```python
from build123d import *

# Parameters (mm, degrees)
SKETCH3_W           = 25.4
SKETCH3_H           = 12.7
SKETCH3_W_2         = 127
BOSS_EXTRUDE1_DEPTH = 6.35
FILLET1_R           = 7.62
SKETCH5_R           = 3.175
CUT_EXTRUDE2_DEPTH  = 13.7


with BuildPart() as part:
    # Sketch3 → Boss-Extrude1 (new body, symmetric)
    with BuildSketch(Plane(origin=(0, 0, 0), x_dir=(0, 0, -1), z_dir=(1, 0, 0))):
        with Locations((88.9, 0)):
            Rectangle(SKETCH3_W, SKETCH3_H)
        Polygon((76.2, 6.35), (50.8, 37.177887789), (50.8, 24.477887789), (65.736097893, 6.35), align=None)
        Polygon((65.736097893, 6.35), (76.2, -6.35), (76.2, 6.35), align=None)
        Polygon((50.8, 37.177887789), (25.4, 6.35), (35.863902107, 6.35), (50.8, 24.477887789), align=None)
        Polygon((35.863902107, 6.35), (25.4, 6.35), (25.4, -6.35), align=None)
        with Locations((-38.1, 0)):
            Rectangle(SKETCH3_W_2, SKETCH3_H)
    extrude(amount=BOSS_EXTRUDE1_DEPTH, both=True)

    # Fillet1
    fillet1_edges = [part.edges().sort_by_distance(p)[0] for p in [
        (0, -6.35, -76.2),
        (0, 24.477887789, -50.8),
        (0, -6.35, -25.4),
        (0, 6.35, -25.4),
        (0, 37.177887789, -50.8),
        (0, 6.35, -76.2),
    ]]
    fillet(fillet1_edges, radius=FILLET1_R)

    # Sketch5 → Cut-Extrude2 (cut, through all)
    with BuildSketch(Plane(origin=(6.35, 0, 0), x_dir=(0, 0, -1), z_dir=(1, 0, 0))):
        with Locations((88.9, 0)):
            Circle(SKETCH5_R)
    extrude(amount=-CUT_EXTRUDE2_DEPTH, mode=Mode.SUBTRACT)


solid = part.part
```
CAD build for the part. Positions are in the model's coordinates, mm. A direction names the side the tool comes from. Coordinates: 2 decimals unless noted, no trailing zeros. Write each loop counter-clockwise with the first axis right and the second up, starting at its lowest first coordinate (ties: lowest second). Pieces come first, ordered by that corner, then holes. Notation, with made-up numbers: (84, -21.5) -> (134, -21.5) arc R18 cw to (134, -15.5) -> close; hole circle Ø6 at (-17, 17.25). An arc over 180 degrees is marked (long way). Use CSV: the item, a comma, the result in double quotes. Start each with the question number.
Item 1: Wall check: probe 1 along Y at (x, z) = (1, -88.9) (3 decimals); probe 2 along Y at (x, z) = (6.25, -80); probe 3 along Z at (x, y) = (0, 1.5). Give the ranges that are in metal, low to high.
Item 2: Band-saw the part on D-D, the plane y = 0. Write the cut outline in (x, z) (3 decimals), plus the area to 3 significant figures.
Item 3: Band-saw the part on A-A, the plane z = -88.9. Write the cut outline in (x, y) (3 decimals), plus the area to 3 significant figures.
Item 4: Tool access for faces 1 (the cylindrical face through (-0.089, -5.641, -76.586)), 2 (the flat face through (0, -6.35, -91)), 3 (the flat face through (0, 6.35, 41)): list every direction of +Z, -Z, +X, -X, +Y, -Y with a clear straight run to the whole face (end or side of a thin tool).
Item 5: Two-plate mould, pull along Z, no slides. Class faces 4 (the flat face through (0, 0, 101.6)), 5 (the cylindrical face through (0.09, 0.14, -85.73)), 6 (the flat face through (0, 6.35, -91)), 7 (the cylindrical face through (-0.089, 20.114, -50.894)): +Z half, -Z half, draft (parallel to the pull), parting line (faces both ways), or undercut.
Item 6: Drop flat-ended pins along their axis: P1, Ø6, axis at y = 17, z = -33, coming from the -X side; P2, Ø6, axis at x = 0.5, y = 29, coming from the -Z side; P3, Ø6.5, axis at x = -3, z = -87.5, coming from the +Y side; P4, Ø4, axis at x = 4, y = 10.5, coming from the -Z side. Give the stop position or say it passes through.
Item 7: Band-saw the part on B-B, the plane y = 12. Write the cut outline in (x, z).
Response values:
1,probe 1,"y = -6.35 to -3.175, 3.175 to 6.35"
1,probe 2,"y = -6.35 to 6.35"
1,probe 3,"z = -101.6 to -91.7, -86.1 to -69.73, -31.87 to 101.6"
2,outline,"(-6.35, -101.6) -> (6.35, -101.6) -> (6.35, -92.075) -> (-6.35, -92.075) -> close; (-6.35, -85.725) -> (6.35, -85.725) -> (6.35, -70.968) -> (-6.35, -70.968) -> close; (-6.35, -30.632) -> (6.35, -30.632) -> (6.35, 101.6) -> (-6.35, 101.6) -> close"
2,area,"1,990 mm2"
3,outline,"(-6.35, -6.35) -> (6.35, -6.35) -> (6.35, -3.175) -> (-6.35, -3.175) -> close; (-6.35, 3.175) -> (6.35, 3.175) -> (6.35, 6.35) -> (-6.35, 6.35) -> close"
3,area,"80.6 mm2"
4,face 1,"+X, -X, -Y"
4,face 2,"+Z, -Z, +X, -X, -Y"
4,face 3,"+Z, +X, -X, +Y"
5,face 4,"+Z half"
5,face 5,"undercut"
5,face 6,"draft"
5,face 7,"undercut"
6,P1,"stops at x = -6.35"
6,P2,"stops at z = -60.01"
6,P3,"stops at y = 6.35"
6,P4,"stops at z = -74.49"
7,outline,"(-6.35, -71.54) -> (6.35, -71.54) -> (6.35, -61.08) -> (-6.35, -61.08) -> close; (-6.35, -40.52) -> (6.35, -40.52) -> (6.35, -30.06) -> (-6.35, -30.06) -> close"
